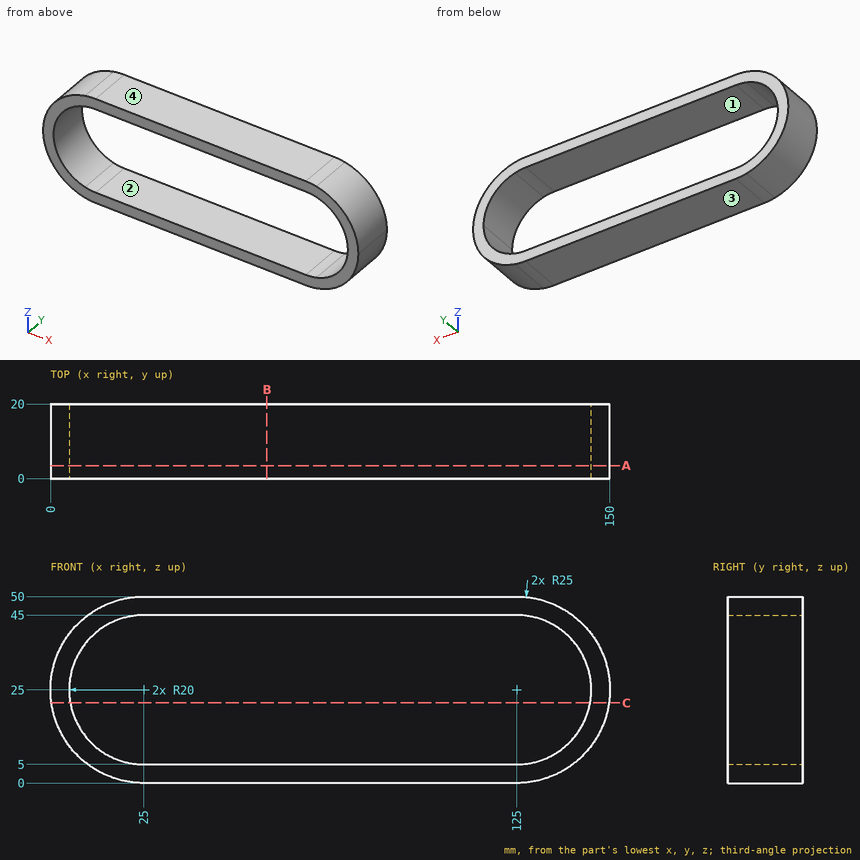
Verification items for this drawing (mm, ordinates from the low corner). Round coordinates to 2 decimals unless told otherwise and drop trailing zeros. Loops run counter-clockwise (first coordinate to the right, second up) from the corner with the lowest first, then second, coordinate; pieces in that order, holes last. Notation, with made-up numbers: (23.5, 52.25) -> (61.5, 52.25) arc R19 cw to (61.5, 56.25) -> close; hole circle Ø2 at (-1.75, 66). An arc over 180 degrees is marked (long way). Answer in a Markdown table with one row per item.
Q1. Release check for a two-part mould opening along Z. For the marked faces 1, 2, 3 and 4 record: released by +Z, released by -Z, zero draft, split by the parting line, or undercut.
Data:
| item | result |
|---|---|
| face 1 | undercut |
| face 2 | undercut |
| face 3 | released by -Z |
| face 4 | released by +Z |
Q2. Thickness scan on L1, parallel to Z at x = 52, y = 6; L2, parallel to X at y = 1.5, z = 43; L3, parallel to X at y = 4.25, z = 19.5. Record the ranges inside material, lowest first.
Data:
| item | result |
|---|---|
| L1 | z = 0 to 5, 45 to 50 |
| L2 | x = 7.65 to 16.28, 133.72 to 142.35 |
| L3 | x = 0.61 to 5.77, 144.23 to 149.39 |
Q3. Go/stop test with flat-tipped pins: P1, Ø6, axis at y = 8.5, z = 8, coming from the -X side; P2, Ø4, axis at y = 13.5, z = 41.5, coming from the +X side; P3, Ø12, axis at y = 5.5, z = 14.5, coming from the -X side. Record where each tip stops, or that it passes through.
Data:
| item | result |
|---|---|
| P1 | stops at x = 4.29 |
| P2 | stops at x = 145.37 |
| P3 | stops at x = 0.41 |
Q4. Sectioned sample at A-A on y = 3.5. Enter the section's corners in (x, z), then the cut area to 3 significant figures.
Data:
| item | result |
|---|---|
| outline | (25, 0) -> (125, 0) arc R25 ccw to (125, 50) -> (25, 50) arc R25 ccw to start; hole (25, 5) -> (125, 5) arc R20 ccw to (125, 45) -> (25, 45) arc R20 ccw to start |
| area | 1,710 mm^2 |
Q5. Sectioned sample at B-B on x = 58. Enter the section's corners in (y, z), then the cut area to 3 significant figures.
Data:
| item | result |
|---|---|
| outline | (0, 0) -> (20, 0) -> (20, 5) -> (0, 5) -> close; (0, 45) -> (20, 45) -> (20, 50) -> (0, 50) -> close |
| area | 200 mm^2 |
Q6. Sectioned sample at C-C on z = 21.5. Enter the section's corners in (x, y), then the cut area to 3 significant figures.
Data:
| item | result |
|---|---|
| outline | (0.25, 0) -> (5.31, 0) -> (5.31, 20) -> (0.25, 20) -> close; (144.69, 0) -> (149.75, 0) -> (149.75, 20) -> (144.69, 20) -> close |
| area | 202 mm^2 |
